Verification items for the finished model (mm, model axes). Face numbers are marked on the shaded views. A direction names the side the tool comes from. Round coordinates to 2 decimals unless told otherwise and drop trailing zeros. Loops run counter-clockwise (first coordinate to the right, second up) from the corner with the lowest first, then second, coordinate; pieces in that order, holes last. Notation, with made-up numbers: M 3.25,18 L 36.25,18 A9 ccw 36.25,35 Z; hole C 87,-17 d10. An arc over 180 degrees is marked long. Answer as CSV lines item,"result".
```python
from build123d import *

# Parameters (mm, degrees)
SKETCH1_R           = 1.75
BOSS_EXTRUDE1_DEPTH = 57.5
BOSS_EXTRUDE2_DEPTH = 8.4
SKETCH3_W           = 5.3
SKETCH3_H           = 35
CUT_EXTRUDE1_DEPTH  = 5.4
CUT_EXTRUDE2_DEPTH  = 85.49881656
SKETCH5_W           = 18.2
SKETCH5_H           = 8.4
SKETCH5_W_2         = 8.4
SKETCH5_H_2         = 8.937392322
SKETCH5_W_3         = 9.875614017
SKETCH5_H_3         = 12.4
CUT_EXTRUDE3_DEPTH  = 18
LPATTERN1_COUNT     = 2
LPATTERN1_PITCH     = 27


with BuildPart() as part:
    # Sketch1 → Boss-Extrude1 (new body)
    with BuildSketch(Plane.XY):
        with BuildLine():
            Line((-52.8, -1.2), (-4.2, -1.2))
            Line((-4.2, -1.2), (-4.2, 0))
            ThreePointArc((-4.2, 0), (0, 4.2), (4.2, 0))
            Line((4.2, 0), (4.2, -1.2))
            Line((4.2, -1.2), (33.3, -1.2))
            Line((33.3, -1.2), (33.3, 0))
            ThreePointArc((33.3, 0), (34.530151519, 2.969848481), (37.5, 4.2))
            Line((37.5, 4.2), (41.5, 4.2))
            Line((41.5, 4.2), (41.5, -4.2))
            Line((41.5, -4.2), (-57, -4.2))
            ThreePointArc((-57, -4.2), (-60.217386661, -2.699707961), (-61.136192563, 0.729322346))
            Line((-61.136192563, 0.729322346), (-59.818910528, 8.2))
            Line((-59.818910528, 8.2), (-57, 8.2))
            Line((-57, 8.2), (-57, 4.2))
            Line((-57, 4.2), (-52.8, 4.2))
            Line((-52.8, 4.2), (-52.8, -1.2))
        make_face()
        Circle(SKETCH1_R, mode=Mode.SUBTRACT)
        with Locations((-57, 0)):
            Circle(SKETCH1_R, mode=Mode.SUBTRACT)
        with Locations((37.5, 0)):
            Circle(SKETCH1_R, mode=Mode.SUBTRACT)
    extrude(amount=BOSS_EXTRUDE1_DEPTH)

    # Sketch2 → Boss-Extrude2 (add)
    with BuildSketch(Plane(origin=(0, 4.2, 0), x_dir=(1, 0, 0), z_dir=(0, 1, 0))):
        Polygon((41.5, -57.5), (51.5, -57.5), (51.5, -17.5), (41.5, 0), align=None)
    extrude(amount=-BOSS_EXTRUDE2_DEPTH)

    # Sketch3 → Cut-Extrude1 (cut)
    with BuildSketch(Plane(origin=(0, 4.2, 0), x_dir=(1, 0, 0), z_dir=(0, 1, 0))):
        with Locations((47.35, -36.75)):
            Rectangle(SKETCH3_W, SKETCH3_H)
    extrude(amount=-CUT_EXTRUDE1_DEPTH, mode=Mode.SUBTRACT)

    # Sketch4 → Cut-Extrude2 (cut, through all)
    with BuildSketch(Plane(origin=(0, -1.2, 0), x_dir=(1, 0, 0), z_dir=(0, 1, 0))):
        with BuildLine():
            Line((-44.921320344, -49.378679656), (-42.8, -47.257359313))
            Line((-42.8, -47.257359313), (-40.678679656, -49.378679656))
            ThreePointArc((-40.678679656, -49.378679656), (-42.8, -54.5), (-44.921320344, -49.378679656))
        make_face()
    cut_extrude2 = extrude(amount=-CUT_EXTRUDE2_DEPTH, mode=Mode.SUBTRACT)

    # Sketch5 → Cut-Extrude3 (cut)
    with BuildSketch(Plane(origin=(0, 0, 0), x_dir=(-1, 0, 0), z_dir=(0, 0, -1))):
        with Locations((-42.4, 0)):
            Rectangle(SKETCH5_W, SKETCH5_H)
        with Locations((0, 0.268696161)):
            Rectangle(SKETCH5_W_2, SKETCH5_H_2)
        with Locations((57.737807008, 2)):
            Rectangle(SKETCH5_W_3, SKETCH5_H_3)
    extrude(amount=-CUT_EXTRUDE3_DEPTH, mode=Mode.SUBTRACT)

    # LPattern1: Cut-Extrude2 ×2
    with Locations(*[(i * LPATTERN1_PITCH, 0, 0) for i in range(1, LPATTERN1_COUNT)]):
        add(cut_extrude2, mode=Mode.SUBTRACT)


solid = part.part
```
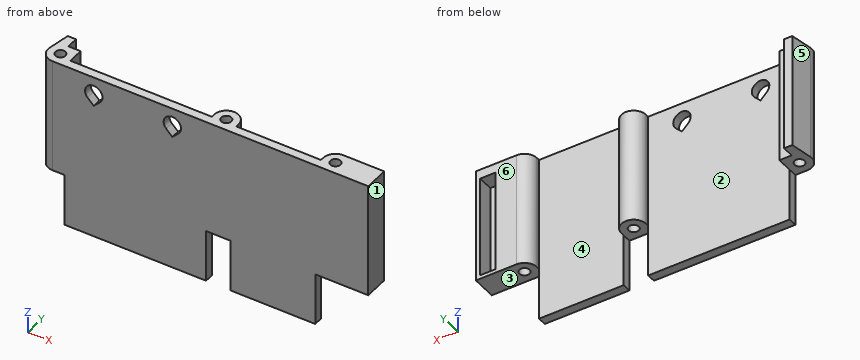
1) Set-up check for the marked faces 4, 5 and 6: record each of +Z, -Z, +X, -X, +Y, -Y from which the full face is reachable in a straight line by a thin tool's end or side.
Here are the results:
face 4,"+Z, -Z, +Y"
face 5,"+Z, -Z, -X, +Y"
face 6,"+Z, -Z, +X, +Y"
2) Go/stop test with flat-tipped pins: pin 1 (1.6 mm diameter, centred on y = 1, z = 34, fed in from -X); pin 2 (8 mm diameter, centred on x = -16.5, z = 14, fed in from +Y); pin 3 (3.5 mm diameter, centred on y = -2, z = 13, fed in from -X). Record where each tip stops, or that it passes through.
Here are the results:
pin 1,"stops at x = -61.2"
pin 2,"stops at y = -1.2"
pin 3,"stops at x = -52.8"
3) Material ranges on probe 1 along X at (y, z) = (0, 19); probe 2 along X at (y, z) = (-2.25, 51.5); probe 3 along Z at (x, y) = (-42.8, -2.45), recorded low to high.
Here are the results:
probe 1,"x = -61.2 to -58.75, -55.25 to -52.8, -4.2 to -1.75, 1.75 to 4.2, 33.3 to 35.75, 39.25 to 51.5"
probe 2,"x = -60.55 to -45.8, -39.8 to -18.8, -12.8 to 51.5"
probe 3,"z = 0 to 47.26, 54.5 to 57.5"
4) Section check B-B (x = 0). Record the cut outline in (y, z).
Here are the results:
outline,"M -4.2,18 L -1.75,18 L -1.75,57.5 L -4.2,57.5 Z; M 1.75,18 L 4.2,18 L 4.2,57.5 L 1.75,57.5 Z"
5) Section check D-D (y = -3). Record the cut outline in (x, z), plus the area to 3 significant figures.
Here are the results:
outline,"M -59.94,18 L -52.8,18 L -52.8,0 L -4.2,0 L -4.2,18 L 4.2,18 L 4.2,0 L 33.3,0 L 33.3,18 L 51.5,18 L 51.5,57.5 L -59.94,57.5 Z; hole M -44.92,49.38 L -42.8,47.26 L -40.68,49.38 A3 ccw long Z; hole M -17.92,49.38 L -15.8,47.26 L -13.68,49.38 A3 ccw long Z"
area,"5,740 mm^2"
6) Section check A-A (z = 51.5). State how many separate pieces and enclosed holes the cut face has, plus the area to 3 significant figures.
Here are the results:
separate pieces,"3"
enclosed holes,"3"
area,"430 mm^2"
7) Section check C-C (z = 7). Record the cut outline in (x, y).
Here are the results:
outline,"M -52.8,-4.2 L -4.2,-4.2 L -4.2,-1.2 L -52.8,-1.2 Z; M 4.2,-4.2 L 33.3,-4.2 L 33.3,-1.2 L 4.2,-1.2 Z"
8) Draft check along X on the marked faces 1, 2 and 3. Enter one of: +X half, -X half, draft (parallel to the pull), parting line (faces both ways), or undercut.
Here are the results:
face 1,"+X half"
face 2,"undercut"
face 3,"draft"
